Build history of the part. All positions in model axes, mm. Face numbers are marked on the shaded views. A direction names the side the tool comes from. Round coordinates to 2 decimals unless told otherwise and drop trailing zeros. Write each loop counter-clockwise with the first axis right and the second up, starting at its lowest first coordinate (ties: lowest second). Pieces come first, ordered by that corner, then holes.
Item 1: Band-saw the part on D-D, the plane y = 20. Count the separate pieces of the cut face and the enclosed holes in it, then the cut area to 3 significant figures.
Item 2: Band-saw the part on B-B, the plane x = 43. Write the cut outline in (y, z).
Item 3: Band-saw the part on A-A, the plane z = 0. Write the cut outline in (x, y).
Item 4: Band-saw the part on C-C, the plane x = 34. Write the cut outline in (y, z), then the cut area to 3 significant figures.
Item 5: Drop flat-ended pins along their axis: pin 1 Ø12 at (y, z) = (22, -0.5) entering from -X; pin 2 Ø10 at (y, z) = (32.5, -22) entering from +X; pin 3 Ø11 at (x, y) = (41, 17.5) entering from +Z; pin 4 Ø13.5 at (x, y) = (34, 19) entering from -Z. Give the stop position or say it passes through.
Item 6: Mould opens along Z. For the marked faces 1, 2 and 3 say: +Z half, -Z half, draft (parallel to the pull), parting line (faces both ways), or undercut.
Item 7: 3-axis set-ups, long thin cutter, end or side, ignore diameter. For the marked faces 4, 5 and 6: which of +Z, -Z, +X, -X, +Y, -Y reach the whole face in a straight line?
Item 8: Wall check: probe 1 along Z at (x, y) = (18, 9); probe 2 along Z at (x, y) = (38, 34); probe 3 along Y at (x, z) = (62, 24). Give the ranges that are in metal, low to high.
```python
from build123d import *

# Parameters (mm, degrees)
SKETCH1_R           = 7.5
BOSS_EXTRUDE1_DEPTH = 29
CUT_EXTRUDE1_DEPTH  = 72
CUT_EXTRUDE2_DEPTH  = 72
SKETCH4_R           = 7
CUT_EXTRUDE3_DEPTH  = 72
CUT_EXTRUDE11_DEPTH = 12
CUT_EXTRUDE12_DEPTH = 6


with BuildPart() as part:
    # Sketch1 → Boss-Extrude1 (new, symmetric)
    with BuildSketch(Plane.XY):
        with BuildLine():
            Line((0, 0), (65, 0))
            Line((65, 0), (80, 8.660254038))
            Line((80, 8.660254038), (80, 31.339745962))
            Line((80, 31.339745962), (65, 40))
            Line((65, 40), (36.66060556, 40))
            ThreePointArc((36.66060556, 40), (16.66060556, 35.82575695), (0, 24))
            Line((0, 24), (0, 0))
        make_face()
        with Locations(Location((34, 19, 0), (0, 0, 180))):
            Circle(SKETCH1_R, mode=Mode.SUBTRACT)
    extrude(amount=BOSS_EXTRUDE1_DEPTH, both=True)

    # Sketch2 → Cut-Extrude1 (cut)
    with BuildSketch(Plane(origin=(0, 0, 0), x_dir=(1, 0, 0), z_dir=(0, 1, 0))):
        Polygon((0, 21), (16, 21), (16, 15), (54, 15), (54, -15), (16, -15), (16, -21), (0, -21), align=None)
    extrude(amount=CUT_EXTRUDE1_DEPTH, mode=Mode.SUBTRACT)

    # Sketch3 → Cut-Extrude2 (cut)
    with BuildSketch(Plane(origin=(0, 0, 0), x_dir=(1, 0, 0), z_dir=(0, 1, 0))):
        Polygon((80, 29), (65, 29), (80, 14), align=None)
        Polygon((65, -29), (80, -29), (80, -14), align=None)
    extrude(amount=CUT_EXTRUDE2_DEPTH, mode=Mode.SUBTRACT)

    # Sketch4 → Cut-Extrude3 (cut)
    with BuildSketch(Plane(origin=(80, 0, 0), x_dir=(0, 0, -1), z_dir=(1, 0, 0))):
        with Locations((0, 20)):
            Circle(SKETCH4_R)
    extrude(amount=-CUT_EXTRUDE3_DEPTH, mode=Mode.SUBTRACT)

    # Sketch6 → Cut-Extrude11 (cut)
    with BuildSketch(Plane.XY.offset(29)):
        with BuildLine():
            Line((63, 2), (63, 38))
            Line((63, 38), (36.66060556, 38))
            ThreePointArc((36.66060556, 38), (27.30122037, 37.078677858), (18.301127214, 34.350079536))
            Line((18.301127214, 34.350079536), (18.301127214, 2))
            Line((18.301127214, 2), (63, 2))
        make_face()
    extrude(amount=-CUT_EXTRUDE11_DEPTH, mode=Mode.SUBTRACT)

    # Sketch8 → Cut-Extrude12 (cut)
    with BuildSketch(Plane.XY.offset(29)):
        with BuildLine():
            Line((0, 2), (18.301127214, 2))
            Line((18.301127214, 2), (18.301127214, 34.350079536))
            ThreePointArc((18.301127214, 34.350079536), (8.350425073, 28.76252934), (0, 20.98386677))
            Line((0, 20.98386677), (0, 2))
        make_face()
    extrude(amount=-CUT_EXTRUDE12_DEPTH, mode=Mode.SUBTRACT)


solid = part.part
```
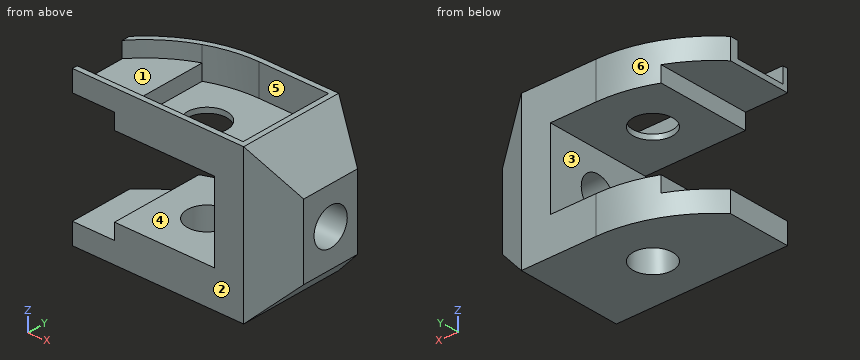
Results:
1. separate pieces: 4
1. enclosed holes: 0
1. area: 1,350 mm2
2. outline: (0, -29) - (40, -29) - (40, -15) - (0, -15) - close; (0, 15) - (40, 15) - (40, 29) - (38, 29) - (38, 17) - (2, 17) - (2, 29) - (0, 29) - close
3. outline: (54, 0) - (65, 0) - (80, 8.66) - (80, 13) - (54, 13) - close; (54, 27) - (80, 27) - (80, 31.34) - (65, 40) - (54, 40) - close
4. outline: (0, -29) - (11.5, -29) - (11.5, -15) - (0, -15) - close; (0, 15) - (11.5, 15) - (11.5, 17) - (2, 17) - (2, 29) - (0, 29) - close; (26.5, -29) - (39.93, -29) - (39.93, -15) - (26.5, -15) - close; (26.5, 15) - (39.93, 15) - (39.93, 29) - (37.93, 29) - (37.93, 17) - (26.5, 17) - close
4. area: 447 mm2
5. pin 1: stops at x = 54
5. pin 2: stops at x = 77
5. pin 3: stops at z = 17
5. pin 4: passes through
6. face 1: +Z half
6. face 2: draft
6. face 3: undercut
7. face 4: -X, +Y, -Y
7. face 5: +Z
7. face 6: +Z, -Z, -X, +Y
8. probe 1: z = -29 to -15, 15 to 23
8. probe 2: z = -29 to -15, 15 to 17
8. probe 3: y = 0 to 2, 38 to 40
